Geometry: see drawing. Coordinates: mm, zero at the bounding-box minimum. Round coordinates to 2 decimals unless told otherwise and drop trailing zeros. Order: outer loops, then holes, each group sorted by start corner. A loop starts at its lowest first (then second) coordinate and runs counter-clockwise, first axis right, second up. Notation, with made-up numbers: (7.5, -24.75) -> (23.5, -24.75) arc R21 cw to (23.5, -15.75) -> close; hole circle Ø9 at (-40, 20). An arc over 180 degrees is marked (long way). Write item = value, one per line. Start each with the question number.
(1) Cut plane B-B on x = 289.5. Return the cut outline in (y, z).
(2) Ray query, line 1 (X direction, y = 68, z = 2.6); line 2 (Y direction, x = 157.5, z = 0.15); line 3 (X direction, y = 39, z = 2.4). Return the intervals inside material, ascending.
(3) Contact query for flat-ended pins moving along their axis: pin 1 Ø0.9 at (y, z) = (36.5, 2) entering from +X; pin 2 Ø0.9 at (x, z) = (2, 1.5) entering from +Y; pin 3 Ø1.5 at (x, z) = (315, 2) entering from +Y. Output: stop coordinate, or through.
(4) Cut plane A-A on z = 1.8. Return the cut outline in (x, y), then the cut area to 3 significant figures.
(5) Cut plane C-C on x = 38. Return the cut outline in (y, z) (1 decimal).
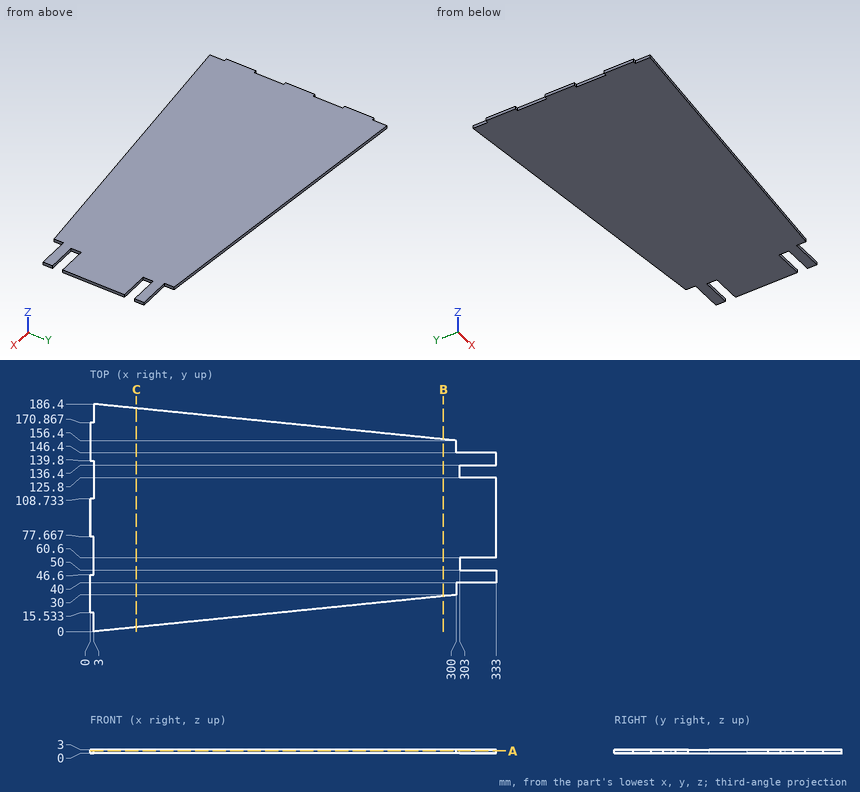
Evaluation:
q1.outline = (28.94, 0) -> (157.46, 0) -> (157.46, 3) -> (28.94, 3) -> close
q2.line_1 = 3 to 333
q2.line_2 = 15.61 to 170.79
q2.line_3 = 0 to 300
q3.pin_1 = 300
q3.pin_2 = 170.87
q3.pin_3 = 146.4
q4.outline = (0, 15.53) -> (3, 15.53) -> (3, 0) -> (300, 30) -> (300, 40) -> (333, 40) -> (333, 50) -> (303, 50) -> (303, 60.6) -> (333, 60.6) -> (333, 125.8) -> (303, 125.8) -> (303, 136.4) -> (333, 136.4) -> (333, 146.4) -> (300, 146.4) -> (300, 156.4) -> (3, 186.4) -> (3, 170.87) -> (0, 170.87) -> (0, 139.8) -> (3, 139.8) -> (3, 108.73) -> (0, 108.73) -> (0, 77.67) -> (3, 77.67) -> (3, 46.6) -> (0, 46.6) -> close
q4.area = 49,600 mm^2
q5.outline = (3.5, 0) -> (182.9, 0) -> (182.9, 3) -> (3.5, 3) -> close
